```python
from build123d import *

# Parameters (mm, degrees)
SKETCH1_R           = 12.62515314
BOSS_EXTRUDE1_DEPTH = 127.254
SKETCH2_W           = 21.600890372
SKETCH2_H           = 6.08719661
CUT_EXTRUDE1_DEPTH  = 155.702
CUT_EXTRUDE2_DEPTH  = 141.081655767
BOSS_EXTRUDE2_DEPTH = 12.755190121
BOSS_EXTRUDE3_DEPTH = 12.755190121
BOSS_EXTRUDE4_DEPTH = 12.7
BOSS_EXTRUDE5_DEPTH = 12.7
SKETCH11_R          = 3.688999931
CUT_EXTRUDE3_DEPTH  = 13.97
SKETCH12_R          = 3.801462188
CUT_EXTRUDE4_DEPTH  = 11.43
SKETCH13_W          = 3.347443601
SKETCH13_H          = 13.720552831
BOSS_EXTRUDE6_DEPTH = 12.7
SKETCH14_W          = 3.264831583
SKETCH14_H          = 12.7
BOSS_EXTRUDE7_DEPTH = 13.97
SKETCH16_R          = 3.69446956
CUT_EXTRUDE6_DEPTH  = 45.212
SKETCH17_R          = 3.700235887
CUT_EXTRUDE7_DEPTH  = 28.702


with BuildPart() as part:
    # Sketch1 → Boss-Extrude1 (new body)
    with BuildSketch(Plane(origin=(0, 0, 0), x_dir=(1, 0, 0), z_dir=(0, 1, 0))):
        with Locations(Location((0, 0, 0), (0, 0, 270))):
            Circle(SKETCH1_R)
    extrude(amount=-BOSS_EXTRUDE1_DEPTH)

    # Sketch2 → Cut-Extrude1 (cut)
    with BuildSketch(Plane(origin=(0, -127.254, 0), x_dir=(-1, 0, 0), z_dir=(0, -1, 0))):
        with Locations((0, -9.581554835)):
            Rectangle(SKETCH2_W, SKETCH2_H)
    extrude(amount=-CUT_EXTRUDE1_DEPTH, mode=Mode.SUBTRACT)

    # Sketch3 → Cut-Extrude2 (cut)
    with BuildSketch(Plane(origin=(0, -127.254, 0), x_dir=(-1, 0, 0), z_dir=(0, -1, 0))):
        with BuildLine():
            Line((3.126169088, 0), (-3.091625783, 0))
            ThreePointArc((-3.091625783, 0), (0.017271652, 3.108897435), (3.126169088, 0))
        make_face()
    extrude(amount=-CUT_EXTRUDE2_DEPTH, mode=Mode.SUBTRACT)

    # Sketch4 → Boss-Extrude2 (add)
    with BuildSketch(Plane.XZ.offset(127.254)):
        Polygon((-10.800445186, 6.53795653), (-8.274777075, 6.53795653), (-10.800445186, 20.396051451), (-13.364649969, 20.396051451), align=None)
    extrude(amount=-BOSS_EXTRUDE2_DEPTH)

    # Sketch5 → Boss-Extrude3 (add)
    with BuildSketch(Plane.XZ.offset(127.254)):
        Polygon((10.800445186, 6.53795653), (8.287884941, 6.53795653), (10.800445186, 20.258509361), (13.265579683, 20.258509361), align=None)
    extrude(amount=-BOSS_EXTRUDE3_DEPTH)

    # Sketch9 → Boss-Extrude4 (add)
    with BuildSketch(Plane(origin=(0, -127.254, 0), x_dir=(-1, 0, 0), z_dir=(0, -1, 0))):
        Polygon((10.800445186, -20.396051451), (8.274777075, -20.396051451), (8.274777075, -6.53795653), align=None)
    extrude(amount=-BOSS_EXTRUDE4_DEPTH)

    # Sketch10 → Boss-Extrude5 (add)
    with BuildSketch(Plane(origin=(0, -127.254, 0), x_dir=(-1, 0, 0), z_dir=(0, -1, 0))):
        Polygon((-8.287884941, -6.53795653), (-8.287884941, -20.258509361), (-10.800445186, -20.258509361), align=None)
    extrude(amount=-BOSS_EXTRUDE5_DEPTH)

    # Sketch11 → Cut-Extrude3 (cut)
    with BuildSketch(Plane.ZY.offset(-8.287884941)):
        with Locations((13.398232945, -120.904)):
            Circle(SKETCH11_R)
    extrude(amount=-CUT_EXTRUDE3_DEPTH, mode=Mode.SUBTRACT)

    # Sketch12 → Cut-Extrude4 (cut)
    with BuildSketch(Plane(origin=(-8.274777075, 0, 0), x_dir=(0, 0, -1), z_dir=(1, 0, 0))):
        with Locations((-13.46700399, -120.904)):
            Circle(SKETCH12_R)
    extrude(amount=-CUT_EXTRUDE4_DEPTH, mode=Mode.SUBTRACT)

    # Sketch13 → Boss-Extrude6 (add)
    with BuildSketch(Plane.XZ.offset(127.254)):
        with Locations((6.614163141, 13.398232946)):
            Rectangle(SKETCH13_W, SKETCH13_H)
    extrude(amount=-BOSS_EXTRUDE6_DEPTH)

    # Sketch14 → Boss-Extrude7 (add)
    with BuildSketch(Plane.XY.offset(20.396051451)):
        with Locations((-6.642361284, -120.904)):
            Rectangle(SKETCH14_W, SKETCH14_H)
    extrude(amount=-BOSS_EXTRUDE7_DEPTH)

    # Sketch16 → Cut-Extrude6 (cut)
    with BuildSketch(Plane.ZY.offset(-4.94044134)):
        with Locations((13.398232945, -120.904)):
            Circle(SKETCH16_R)
    extrude(amount=-CUT_EXTRUDE6_DEPTH, mode=Mode.SUBTRACT)

    # Sketch17 → Cut-Extrude7 (cut)
    with BuildSketch(Plane(origin=(-5.009945492, 0, 0), x_dir=(0, 0, -1), z_dir=(1, 0, 0))):
        with Locations((-13.46700399, -120.904)):
            Circle(SKETCH17_R)
    extrude(amount=-CUT_EXTRUDE7_DEPTH, mode=Mode.SUBTRACT)


solid = part.part
```
Here's how the part is built. I have some questions about the finished solid (model axes, mm). A direction names the side the tool comes from. Round coordinates to 2 decimals unless told otherwise and drop trailing zeros. Loops run counter-clockwise (first coordinate to the right, second up) from the corner with the lowest first, then second, coordinate; pieces in that order, holes last.
1. Will these pins go through, and if not, where does the flat tip stop? pin 1 (5 mm diameter, centred on x = -5.5, z = 4.5, fed in from +Y); pin 2 (6.5 mm diameter, centred on x = 8.5, z = 13, fed in from +Y); pin 3 (10 mm diameter, centred on y = -120.9, z = 13.47, fed in from -X); pin 4 (5 mm diameter, centred on y = -21.5, z = 4, fed in from +X).
Answers:
pin 1: stops at y = 0
pin 2: stops at y = -114.5
pin 3: stops at x = -13.01
pin 4: stops at x = 12.54
2. Suppose I cut it at C-C, the plane z = 8. Please give me the cut outline in (x, y), and give its area (3 significant figures).
Answers:
outline: (-11.07, -127.25) - (-5.01, -127.25) - (-5.01, -114.55) - (-8.54, -114.55) - (-8.54, -114.5) - (-11.07, -114.5) - close; (4.94, -127.25) - (11.06, -127.25) - (11.06, -114.5) - (8.56, -114.5) - (8.56, -114.55) - (4.94, -114.55) - close
area: 155 mm2
3. If I drill on probe 1 along Y at (x, z) = (-10.25, 13.5); probe 2 along Z at (x, y) = (1, -80); probe 3 along Z at (x, y) = (6.5, -17), over which ranges is the centre line in solid material (lowest first)?
Answers:
probe 1: y = -127.25 to -124.71, -117.1 to -114.5
probe 2: z = -12.59 to -2.94, 0 to 6.54
probe 3: z = -10.82 to 6.54
4. Suppose I cut it at D-D, the plane y = -90. Please give me the cut outline in (x, z), and give its area (3 significant figures).
Answers:
outline: (-10.8, 6.54) arc R12.63 ccw (long way) to (10.8, 6.54) - close; hole (-3.13, 0) arc R3.11 ccw to (3.09, 0) - close
area: 393 mm2
5. Thinking about a two-plate mould opening in Y: for faces 6 (the face through (8.76, -119.79, 16.92)), 7 (the face through (-11.53, -123.8, 10.48)), 8 (the face through (-7, -114.554, 14)), which applies, released by +Y, released by -Y, zero draft, split by the parting line, or undercut?
Answers:
face 6: undercut
face 7: zero draft
face 8: released by +Y
6. Suppose I cut it at A-A, the plane y = -118.5. Please give me the cut outline in (x, z), and give its area (3 significant figures).
Answers:
outline: (-13.36, 20.4) - (-12.63, 16.41) - (-8.27, 16.41) - (-8.27, 16.28) - (-5.01, 16.28) - (-5.01, 20.4) - close; (-11.54, 10.52) - (-10.8, 6.54) arc R12.63 ccw (long way) to (10.8, 6.54) - (11.53, 10.59) - (4.94, 10.59) - (4.94, 6.54) - (-5.01, 6.54) - (-5.01, 10.65) - (-8.27, 10.65) - (-8.27, 10.52) - close; (4.94, 16.2) - (12.54, 16.2) - (13.27, 20.26) - (4.94, 20.26) - close; hole (-3.13, 0) arc R3.11 ccw to (3.09, 0) - close
area: 507 mm2
7. Suppose I cut it at B-B, the plane x = 0. Please give me the cut outline in (y, z).
Answers:
outline: (-127.25, -12.63) - (0, -12.63) - (0, -3.11) - (-127.25, -3.11) - close; (-127.25, 0) - (0, 0) - (0, 6.54) - (-127.25, 6.54) - close
8. For faces 1 (the face through (12.598, -123.8, 16.543)), 2 (the face through (-5.01, -118, 10)), 3 (the face through (0, -65, 0)), 4 (the face through (-10.023, -120.737, 17.265)), 5 (the face through (9, -121, 20.259)), which set-ups out of +Z, -Z, +X, -X, +Y, -Y let a thin tool reach every point of the face, with its end or its side?
Answers:
face 1: +X, +Y, -Y
face 2: +Z, +Y, -Y
face 3: +Y, -Y
face 4: -X
face 5: +Z, +X, +Y, -Y
